Could you check a few things on this model? Use its own coordinates, in mm. A direction names the side the tool comes from. Coordinates: 2 decimals unless noted, no trailing zeros. Order: outer loops, then holes, each group sorted by start corner. A loop starts at its lowest first (then second) coordinate and runs counter-clockwise, first axis right, second up. Notation, with made-up numbers: (59, -34) -> (95, -34) arc R32 cw to (95, 5) -> close; hole circle Ø9 at (16, 54). An arc over 180 degrees is marked (long way). Use a Markdown table: item, result. Add a question column.
1) Will these pins go through, and if not, where does the flat tip stop? pin 1 Ø5 at (x, y) = (23, 24) entering from +Z; pin 2 Ø14.5 at (x, y) = (21.5, 35.5) entering from +Z; pin 3 Ø3 at (x, z) = (9, 8) entering from +Y (3 decimals); pin 4 Ø1.8 at (x, y) = (3, 3.115) entering from -Z.
2) If I drill on L1, parallel to Y at x = 14.25, z = 3.5 (3 decimals); L2, parallel to Y at x = 26, z = 1.9 (3 decimals); L3, parallel to X at y = 36, z = 3.75, over which ranges is the centre line in solid material (lowest first)? Write a range as [from, to].
3) If we section it at A-A (y = 39): Write out the boundary of the cut face in (x, z).
4) Thinking about a two-plate mould opening in X: for faces 1 (the flat face through (23, 5, 11)), 2 (the flat face through (14, 55.5, 2)), 3 (the flat face through (6, 5, 11)), 4 (the flat face through (2, 18, 3)), which applies, +X half, -X half, draft (parallel to the pull), parting line (faces both ways), or undercut?
5) If we section it at B-B (x = 9.25): Write out the boundary of the cut face in (y, z) (3 decimals).
6) Which directions (+Z, -Z, +X, -X, +Y, -Y) give clear straight access to the entire face, cutting with the end or side of a thin tool? Please do faces 5 (the cylindrical face through (14.3, 53, 2)), 6 (the cylindrical face through (2.601, 30.545, 2.986)), 7 (the flat face through (29, 27, 2)).
7) If we section it at D-D (x = 15.5): Write out the boundary of the cut face in (y, z) (3 decimals).
8) If we section it at C-C (y = 20.5): Write out the boundary of the cut face in (x, z).
```python
from build123d import *

# Parameters (mm, degrees)
SKETCH1_W             = 29
SKETCH1_H             = 55.5
BODY_DEPTH            = 4
SKETCH2_R             = 1.5
BOLT_HOLES_DEPTH      = 5
SERVO_CLEARANCE_DEPTH = 5
SKETCH4_W             = 25
SKETCH4_H             = 25
FAN_RECESS_DEPTH      = 2
CLAMP_FILLETS_R       = 1
FAN_FILLETS_R         = 2
SKETCH5_W             = 17
SKETCH5_H             = 2
CLAMP_BASE_DEPTH      = 8.25
CLAMP_HOOK_DEPTH      = 17


with BuildPart() as part:
    # Sketch1 → Body (new body)
    with BuildSketch(Plane.XY):
        with Locations((14.5, 27.75)):
            Rectangle(SKETCH1_W, SKETCH1_H)
    extrude(amount=BODY_DEPTH)

    # Sketch2 → Bolt Holes (cut, through all)
    with BuildSketch(Plane.XY.offset(4)):
        with Locations((3, 52.385)):
            Circle(SKETCH2_R)
        with Locations((26, 52.385)):
            Circle(SKETCH2_R)
        with Locations((26, 3.115)):
            Circle(SKETCH2_R)
        with Locations((3, 3.115)):
            Circle(SKETCH2_R)
    extrude(amount=-BOLT_HOLES_DEPTH, mode=Mode.SUBTRACT)

    # Sketch3 → Servo Clearance (cut, through all)
    with BuildSketch(Plane.XY.offset(4)):
        with BuildLine():
            Line((4.5, 12.5898827), (4.5, 8.615))
            Line((4.5, 8.615), (24.5, 8.615))
            Line((24.5, 8.615), (24.5, 12.5898827))
            ThreePointArc((24.5, 12.5898827), (26.69, 16), (24.5, 19.4101173))
            Line((24.5, 19.4101173), (24.5, 28.615))
            Line((24.5, 28.615), (4.5, 28.615))
            Line((4.5, 28.615), (4.5, 19.4101173))
            ThreePointArc((4.5, 19.4101173), (2.31, 16), (4.5, 12.5898827))
        make_face()
        with BuildLine():
            Line((2, 47), (5.33484861, 47))
            ThreePointArc((5.33484861, 47), (14.5, 53), (23.66515139, 47))
            Line((23.66515139, 47), (27, 47))
            Line((27, 47), (27, 33))
            Line((27, 33), (2, 33))
            Line((2, 33), (2, 47))
        make_face()
    extrude(amount=-SERVO_CLEARANCE_DEPTH, mode=Mode.SUBTRACT)

    # Sketch4 → Fan Recess (cut)
    with BuildSketch(Plane.XY.offset(4)):
        with Locations((14.5, 18.615)):
            Rectangle(SKETCH4_W, SKETCH4_H)
    extrude(amount=-FAN_RECESS_DEPTH, mode=Mode.SUBTRACT)

    # Clamp Fillets
    clamp_fillets_edges = [part.edges().sort_by_distance(p)[0] for p in [
        (4.5, 28.615, 1),
        (24.5, 28.615, 1),
        (24.5, 8.615, 1),
        (4.5, 8.615, 1),
        (2, 33, 2),
        (2, 47, 2),
        (5.33484861, 47, 2),
        (23.66515139, 47, 2),
        (27, 47, 2),
        (27, 33, 2),
        (0, 55.5, 2),
        (29, 55.5, 2),
        (29, 0, 2),
        (0, 0, 2),
    ]]
    fillet(clamp_fillets_edges, radius=CLAMP_FILLETS_R)

    # Fan Fillets
    fan_fillets_edges = [part.edges().sort_by_distance(p)[0] for p in [
        (27, 6.115, 3),
        (27, 31.115, 3),
        (2, 31.115, 3),
        (2, 6.115, 3),
    ]]
    fillet(fan_fillets_edges, radius=FAN_FILLETS_R)

    # Sketch5 → Clamp Base (add)
    with BuildSketch(Plane.XY.offset(4)):
        with Locations((14.5, 5.115)):
            Rectangle(SKETCH5_W, SKETCH5_H)
    extrude(amount=CLAMP_BASE_DEPTH)

    # Sketch7 → Clamp Hook (add)
    with BuildSketch(Plane.ZY.offset(-6)):
        Polygon((12.25, 4.115), (15.25, 4.115), (15.25, 6.115), (13.25, 8.115), (12.25, 8.115), align=None)
    extrude(amount=-CLAMP_HOOK_DEPTH)


solid = part.part
```
Answer sheet:
| question | item | result |
|---|---|---|
| 1 | pin 1 | z = 2 |
| 1 | pin 2 | z = 4 |
| 1 | pin 3 | y = 6.115 |
| 1 | pin 4 | through |
| 2 | L1 | [0, 6.115], [31.115, 33], [52.997, 55.5] |
| 2 | L2 | [0, 1.615], [4.615, 13.832], [18.168, 33], [47, 50.885], [53.885, 55.5] |
| 2 | L3 | [0, 2], [27, 29] |
| 3 | outline | (0, 0) -> (2, 0) -> (2, 4) -> (0, 4) -> close; (27, 0) -> (29, 0) -> (29, 4) -> (27, 4) -> close |
| 4 | face 1 | +X half |
| 4 | face 2 | draft |
| 4 | face 3 | -X half |
| 4 | face 4 | undercut |
| 5 | outline | (0, 0) -> (8.615, 0) -> (8.615, 2) -> (6.115, 2) -> (6.115, 12.25) -> (8.115, 12.25) -> (8.115, 13.25) -> (6.115, 15.25) -> (4.115, 15.25) -> (4.115, 4) -> (0, 4) -> close; (28.615, 0) -> (33, 0) -> (33, 4) -> (31.115, 4) -> (31.115, 2) -> (28.615, 2) -> close; (51.511, 0) -> (55.5, 0) -> (55.5, 4) -> (51.511, 4) -> close |
| 6 | face 5 | +Z, -Z |
| 6 | face 6 | +Z |
| 6 | face 7 | +Z, -Z, +X, +Y, -Y |
| 7 | outline | (0, 0) -> (8.615, 0) -> (8.615, 2) -> (6.115, 2) -> (6.115, 12.25) -> (8.115, 12.25) -> (8.115, 13.25) -> (6.115, 15.25) -> (4.115, 15.25) -> (4.115, 4) -> (0, 4) -> close; (28.615, 0) -> (33, 0) -> (33, 4) -> (31.115, 4) -> (31.115, 2) -> (28.615, 2) -> close; (52.95, 0) -> (55.5, 0) -> (55.5, 4) -> (52.95, 4) -> close |
| 8 | outline | (0, 0) -> (4.5, 0) -> (4.5, 2) -> (2, 2) -> (2, 4) -> (0, 4) -> close; (24.5, 0) -> (29, 0) -> (29, 4) -> (27, 4) -> (27, 2) -> (24.5, 2) -> close |
